Geometry check sheet. Reference: the model listing, model coordinates, mm. Face numbers are marked on the shaded views. A direction names the side the tool comes from. Round coordinates to 2 decimals unless told otherwise and drop trailing zeros. Write each loop counter-clockwise with the first axis right and the second up, starting at its lowest first coordinate (ties: lowest second). Pieces come first, ordered by that corner, then holes. Notation, with made-up numbers: (53, -15.75) -> (78, -15.75) arc R24 ccw to (78, 9.25) -> close; hole circle Ø7 at (24, -4). An arc over 180 degrees is marked (long way). Use a Markdown table: item, result.
```python
from build123d import *

# Parameters (mm, degrees)
SKETCH_1_W          = 40
SKETCH_1_H          = 20
EXTRUDE_1_DEPTH     = 10
SKETCH_2_W          = 50
SKETCH_2_H          = 30
EXTRUDE_2_DEPTH     = 5
FILLET_1_R          = 1
SKETCH_3_R          = 1.5
CUT_EXTRUDE_1_DEPTH = 33.787192622


with BuildPart() as part:
    # 草图1 → 凸台-拉伸1 (new body)
    with BuildSketch(Plane.XY):
        Rectangle(SKETCH_1_W, SKETCH_1_H)
    extrude(amount=EXTRUDE_1_DEPTH)

    # 草图2 → 凸台-拉伸2 (add)
    with BuildSketch(Plane.XY.offset(10)):
        Rectangle(SKETCH_2_W, SKETCH_2_H)
    extrude(amount=EXTRUDE_2_DEPTH)

    # 圆角1
    fillet_1_edges = [part.edges().sort_by_distance(p)[0] for p in [
        (-20, 0, 10),
        (0, -10, 10),
        (25, 0, 10),
        (25, -15, 12.5),
        (0, 15, 10),
        (25, 15, 12.5),
        (-25, 0, 10),
        (-25, 15, 12.5),
        (0, -15, 10),
        (-25, -15, 12.5),
        (25, 0, 15),
        (0, 15, 15),
        (-25, 0, 15),
        (0, -15, 15),
        (20, 0, 10),
        (0, -10, 0),
        (-20, 0, 0),
        (0, 10, 0),
        (20, 0, 0),
        (0, 10, 10),
        (20, -10, 5),
        (-20, -10, 5),
        (-20, 10, 5),
        (20, 10, 5),
    ]]
    fillet(fillet_1_edges, radius=FILLET_1_R)

    # 草图3 → 切除-拉伸1 (cut, through all)
    with BuildSketch(Plane(origin=(0, 0, 0), x_dir=(-1, 0, 0), z_dir=(0, 0, -1))):
        with Locations((-4.518689194, -2.140431724)):
            Circle(SKETCH_3_R)
        with Locations((4.518689194, 2.140431724)):
            Circle(SKETCH_3_R)
        with Locations((-4.518689194, 2.140431724)):
            Circle(SKETCH_3_R)
        with Locations((4.518689194, -2.140431724)):
            Circle(SKETCH_3_R)
    extrude(amount=-CUT_EXTRUDE_1_DEPTH, mode=Mode.SUBTRACT)


solid = part.part
```
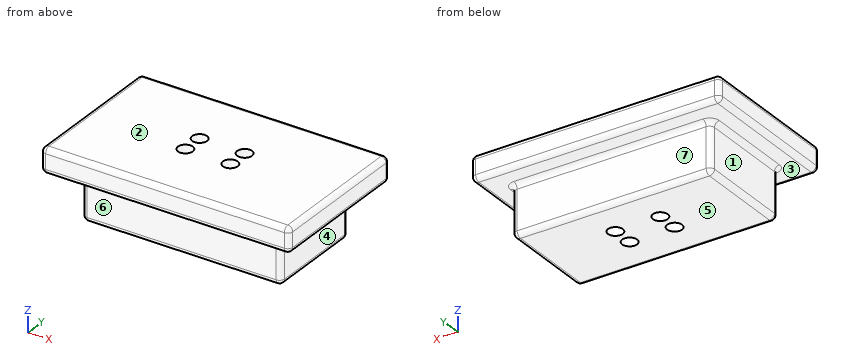
(1) Thickness scan on line 1 (X direction, y = -1, z = 4.5); line 2 (Y direction, x = -4, z = 3.25); line 3 (X direction, y = -3.5, z = 5) (3 decimals). Record the ranges inside material, lowest first.
A:
| item | result |
|---|---|
| line 1 | x = -20 to -5.49, -3.54 to 3.54, 5.49 to 20 |
| line 2 | y = -10 to -3.55, -0.73 to 0.73, 3.55 to 10 |
| line 3 | x = -20 to -5.152, -3.885 to 3.885, 5.152 to 20 |
(2) Section check A-A on x = -4.5. Record the cut outline in (y, z), plus the area to 3 significant figures.
A:
| item | result |
|---|---|
| outline | (-15, 11) arc R1 ccw to (-14, 10) -> (-11, 10) arc R1 cw to (-10, 9) -> (-10, 1) arc R1 ccw to (-9, 0) -> (-3.64, 0) -> (-3.64, 15) -> (-14, 15) arc R1 ccw to (-15, 14) -> close; (-0.64, 0) -> (0.64, 0) -> (0.64, 15) -> (-0.64, 15) -> close; (3.64, 0) -> (9, 0) arc R1 ccw to (10, 1) -> (10, 9) arc R1 cw to (11, 10) -> (14, 10) arc R1 ccw to (15, 11) -> (15, 14) arc R1 ccw to (14, 15) -> (3.64, 15) -> close |
| area | 259 mm2 |
(3) Gauge pin test, flat ends, axial feed: pin 1 Ø5 at (x, y) = (-4.52, 2.14) entering from +Z; pin 2 Ø1 at (x, z) = (13, 7) entering from -Y; pin 3 Ø9 at (x, z) = (-7, 4.5) entering from +Y; pin 4 Ø2.5 at (y, z) = (2, 3.5) entering from -X. Record the tip position at first contact, or that the pin passes through.
A:
| item | result |
|---|---|
| pin 1 | stops at z = 15 |
| pin 2 | stops at y = -10 |
| pin 3 | stops at y = 10 |
| pin 4 | stops at x = -20 |
(4) Release check for a two-part mould opening along Y. For the marked faces 5, 6 and 7 record: +Y half, -Y half, draft (parallel to the pull), parting line (faces both ways), or undercut.
A:
| item | result |
|---|---|
| face 5 | draft |
| face 6 | -Y half |
| face 7 | +Y half |
(5) Section check C-C on z = 12.25. Record the cut outline in (x, y), plus the area to 3 significant figures.
A:
| item | result |
|---|---|
| outline | (-25, -14) arc R1 ccw to (-24, -15) -> (24, -15) arc R1 ccw to (25, -14) -> (25, 14) arc R1 ccw to (24, 15) -> (-24, 15) arc R1 ccw to (-25, 14) -> close; hole circle Ø3 at (-4.52, -2.14); hole circle Ø3 at (-4.52, 2.14); hole circle Ø3 at (4.52, -2.14); hole circle Ø3 at (4.52, 2.14) |
| area | 1,470 mm2 |
(6) Section check B-B on y = -6.25. Record the cut outline in (x, z).
A:
| item | result |
|---|---|
| outline | (-25, 11) arc R1 ccw to (-24, 10) -> (-21, 10) arc R1 cw to (-20, 9) -> (-20, 1) arc R1 ccw to (-19, 0) -> (19, 0) arc R1 ccw to (20, 1) -> (20, 9) arc R1 cw to (21, 10) -> (24, 10) arc R1 ccw to (25, 11) -> (25, 14) arc R1 ccw to (24, 15) -> (-24, 15) arc R1 ccw to (-25, 14) -> close |
(7) Access from +Z, -Z, +X, -X, +Y, -Y to the whole of each face (thin tool, end or side, straight path). Record for the marked faces 1, 2, 3 and 4.
A:
| item | result |
|---|---|
| face 1 | -Z, -X, +Y, -Y |
| face 2 | +Z, +X, -X, +Y, -Y |
| face 3 | -Z |
| face 4 | -Z, +X, +Y, -Y |
(8) Section check D-D on x = -22. Record the cut outline in (y, z).
A:
| item | result |
|---|---|
| outline | (-15, 11) arc R1 ccw to (-14, 10) -> (14, 10) arc R1 ccw to (15, 11) -> (15, 14) arc R1 ccw to (14, 15) -> (-14, 15) arc R1 ccw to (-15, 14) -> close |
